Can you work these out from the drawing? Everything is in mm from the part's minimum corner. Round coordinates to 2 decimals unless told otherwise and drop trailing zeros. Write each loop counter-clockwise with the first axis right and the second up, starting at its lowest first coordinate (ties: lowest second). Pieces come first, ordered by that corner, then holes. Notation, with made-up numbers: (-18.75, 29.25) - (35.25, 29.25) arc R4 cw to (35.25, 33.25) - close; hole circle Ø9 at (7.5, 82.25). An arc over 180 degrees is marked (long way). Write each question's results on one line, items separated by ' | '. Start each with the question number.
(1) Imagine slicing it at B-B on y = 22.5. Write out the boundary of the cut face in (x, z) (1 decimal).
(2) For P1, Ø0.8, axis at x = 19.5, z = 1, coming from the -Y side; P2, Ø0.8, axis at x = 19.5, z = 0.5, coming from the +Y side, each with a flat end and sliding along its axis, tell me the tip position at first contact or that it passes through.
(3) Imagine slicing it at D-D on y = 12. Write out the boundary of the cut face in (x, z).
(4) Please list where these lines run through material, in increasing order: line 1 (X direction, y = 15, z = 0.8) (1 decimal); line 2 (Y direction, x = 16, z = 0.1) (1 decimal); line 3 (X direction, y = 14, z = 0.4) (1 decimal). Write a range as [from, to].
(5) Imagine slicing it at C-C on z = 0.7. Write out the boundary of the cut face in (x, y).
(6) Imagine slicing it at A-A on x = 19.05. Write out the boundary of the cut face in (y, z).
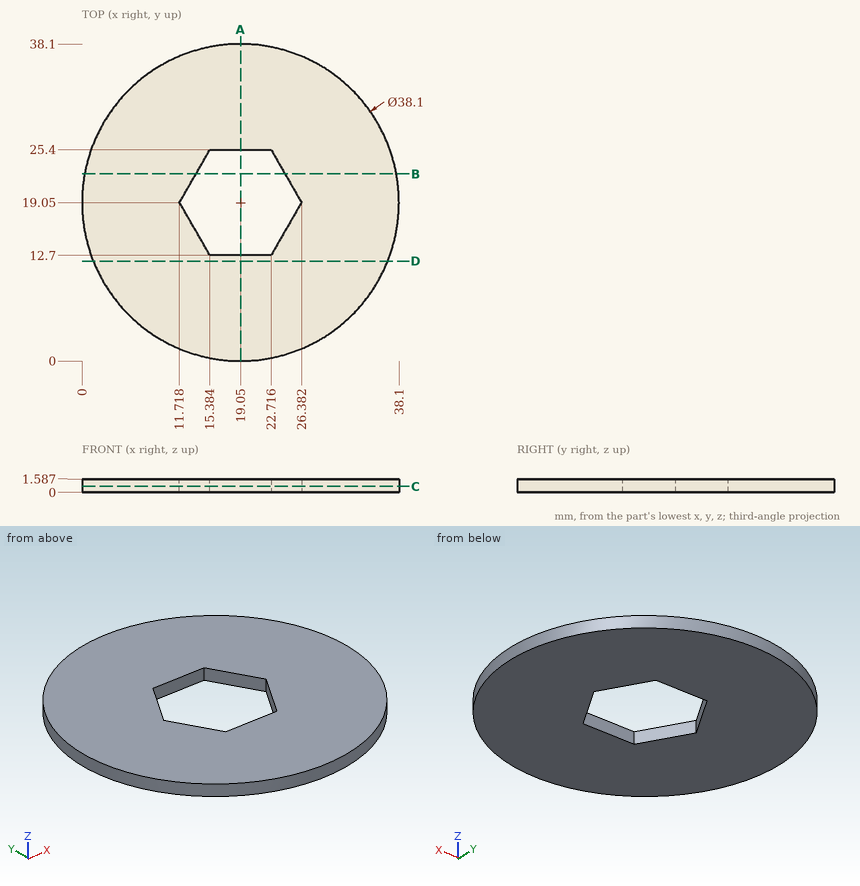
Response:
1) outline: (0.3, 0) - (13.7, 0) - (13.7, 1.6) - (0.3, 1.6) - close; (24.4, 0) - (37.8, 0) - (37.8, 1.6) - (24.4, 1.6) - close
2) P1: y = 0 | P2: y = 38.1
3) outline: (1.35, 0) - (36.75, 0) - (36.75, 1.59) - (1.35, 1.59) - close
4) line 1: [0.4, 14.1], [24, 37.7] | line 2: [0.2, 12.7], [25.4, 37.9] | line 3: [0.7, 14.6], [23.5, 37.4]
5) outline: circle Ø38.1 at (19.05, 19.05); hole (11.72, 19.05) - (15.38, 12.7) - (22.72, 12.7) - (26.38, 19.05) - (22.72, 25.4) - (15.38, 25.4) - close
6) outline: (0, 0) - (12.7, 0) - (12.7, 1.59) - (0, 1.59) - close; (25.4, 0) - (38.1, 0) - (38.1, 1.59) - (25.4, 1.59) - close
